Model file for the job. Use its own axes, mm. Face numbers are marked on the shaded views. A direction names the side the tool comes from. Give positions to 0.01 mm unless a question says otherwise; leave off trailing zeros. Loops run counter-clockwise (first coordinate to the right, second up) from the corner with the lowest first, then second, coordinate; pieces in that order, holes last. Notation, with made-up numbers: M 28.25,-22.75 L 43.25,-22.75 A27 ccw 43.25,2.25 Z; hole C 26,36.5 d3. An arc over 180 degrees is marked long. Answer in a Markdown table with one row per item.
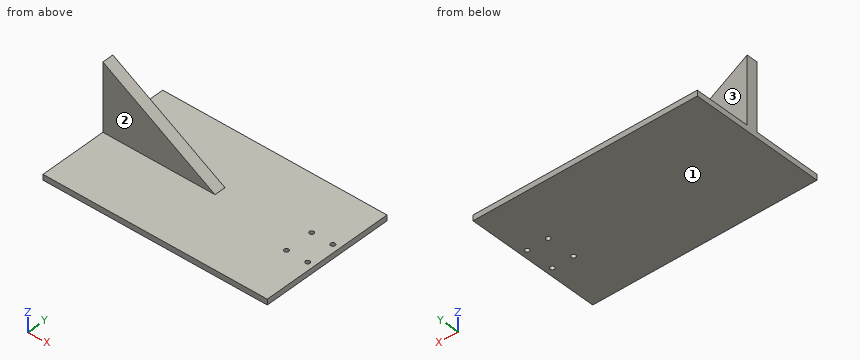
```python
from build123d import *

# Parameters (mm, degrees)
ESQUISSE1_W             = 127
ESQUISSE1_H             = 76.2
BOSS_EXTRU_1_DEPTH      = 1.5875
ESQUISSE2_R             = 1.24968
ENL_V_MAT_EXTRU_1_DEPTH = 75.121121315
BOSS_EXTRUDE1_DEPTH     = 6.35


with BuildPart() as part:
    # Esquisse1 → Boss.-Extru.1 (new, symmetric)
    with BuildSketch(Plane.XY):
        Rectangle(ESQUISSE1_W, ESQUISSE1_H)
    extrude(amount=BOSS_EXTRU_1_DEPTH, both=True)

    # Esquisse2 → Enlèv. mat.-Extru.1 (cut, through all)
    with BuildSketch(Plane.XY.offset(1.5875)):
        with Locations((47.625, 8)):
            Circle(ESQUISSE2_R)
        with Locations((59.625, 8)):
            Circle(ESQUISSE2_R)
    enl_v_mat_extru_1 = extrude(amount=-ENL_V_MAT_EXTRU_1_DEPTH, mode=Mode.SUBTRACT)

    # Symétrie1: Enlèv. mat.-Extru.1 across plane
    add(enl_v_mat_extru_1.mirror(Plane.ZX), mode=Mode.SUBTRACT)

    # Sketch1 → Boss-Extrude1 (add)
    with BuildSketch(Plane(origin=(0, 0, 0), x_dir=(1, 0, 0), z_dir=(0, 1, 0))):
        Polygon((-63.5, -1.5875), (-63.5, -39.6875), (0, -1.5875), align=None)
    extrude(amount=BOSS_EXTRUDE1_DEPTH)


solid = part.part
```
(1) Which spindle directions (+Z, -Z, +X, -X, +Y, -Y) get a long thin tool onto all of the face, cutting with end or side? Do the marked faces 1, 2 and 3. Say none if no direction does.
Established:
| item | result |
|---|---|
| face 1 | -Z, +X, -X, +Y, -Y |
| face 2 | +Z, +X, -X, -Y |
| face 3 | +Z, +X, -X, +Y |
(2) Saw through at B-B, the plane x = 39. Give the cut face in (y, z).
Established:
| item | result |
|---|---|
| outline | M -38.1,-1.59 L 38.1,-1.59 L 38.1,1.59 L -38.1,1.59 Z |
(3) Saw through at A-A, the plane y = 8. Give the cut face in (x, z), and give its area (3 significant figures).
Established:
| item | result |
|---|---|
| outline | M -63.5,-1.59 L 46.38,-1.59 L 46.38,1.59 L -63.5,1.59 Z; M 48.87,-1.59 L 58.38,-1.59 L 58.38,1.59 L 48.87,1.59 Z; M 60.87,-1.59 L 63.5,-1.59 L 63.5,1.59 L 60.87,1.59 Z |
| area | 387 mm2 |
(4) Flat gauge pins, fed straight in: P1, Ø4, axis at x = 47.625, y = -8, coming from the +Z side; P2, Ø3, axis at x = -33, z = 16, coming from the -Y side. Where does each tip first touch, or does it go through?
Established:
| item | result |
|---|---|
| P1 | stops at z = 1.59 |
| P2 | stops at y = 0 |
(5) Saw through at C-C, the plane z = 16.5. Give the cut face in (x, y).
Established:
| item | result |
|---|---|
| outline | M -63.5,0 L -24.85,0 L -24.85,6.35 L -63.5,6.35 Z |
(6) Wall check: L1, parallel to X at y = -8, z = 0.6; L2, parallel to Y at x = -10, z = 7; L3, parallel to Z at x = -11, y = -19.5. Give the ranges that are in metal, low to high.
Established:
| item | result |
|---|---|
| L1 | x = -63.5 to 46.38, 48.87 to 58.38, 60.87 to 63.5 |
| L2 | y = 0 to 6.35 |
| L3 | z = -1.59 to 1.59 |
